Geometry: final body of the model. Coordinates: model frame, mm. Face numbers are marked on the shaded views. A direction names the side the tool comes from. Round coordinates to 2 decimals unless told otherwise and drop trailing zeros. Loops run counter-clockwise (first coordinate to the right, second up) from the corner with the lowest first, then second, coordinate; pieces in that order, holes last. Notation, with made-up numbers: (65, -27.5) -> (110, -27.5) arc R33 ccw to (110, 0.5) -> close; hole circle Ø9 at (18, 65.5). An arc over 180 degrees is marked (long way). Answer in a Markdown table with one row per item.
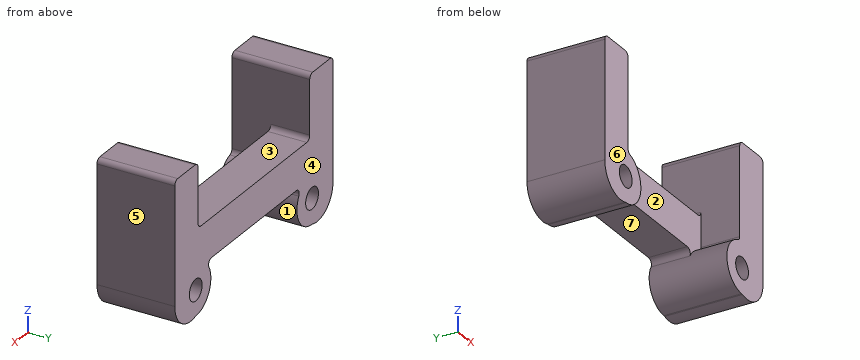
```python
from build123d import *

# Parameters (mm, degrees)
SKETCH1_R           = 1.1
BASE_DEPTH          = 8
BOSS_EXTRUDE2_START = -4
BOSS_EXTRUDE2_DEPTH = 4
FILLET1_R           = 0.5


with BuildPart() as part:
    # Sketch1 → Base (new body)
    with BuildSketch(Plane(origin=(0, 0, 0), x_dir=(1, 0, 0), z_dir=(0, 1, 0))):
        with BuildLine():
            Line((3.6, 0), (3.6, -12.569046516))
            Line((3.6, -12.569046516), (-0.4, -12.569046516))
            Line((-0.4, -12.569046516), (-0.4, -2.569046516))
            ThreePointArc((-0.4, -2.569046516), (-2.592250079, 0.20059793), (0, 2.6))
            ThreePointArc((0, 2.6), (2.464704684, 2.220360331), (3.6, 0))
        make_face()
        with Locations(Location((0, 0, 0), (0, 0, 270))):
            Circle(SKETCH1_R, mode=Mode.SUBTRACT)
    extrude(amount=BASE_DEPTH)

    # Sketch2 → Boss-Extrude2 (add)
    with BuildSketch(Plane(origin=(0, 8, 0), x_dir=(1, 0, 0), z_dir=(0, 1, 0)).offset(BOSS_EXTRUDE2_START)):
        with BuildLine():
            ThreePointArc((-0.4, -2.569046516), (-1.069213935, -2.369975013), (-1.661324773, -2))
            Line((-1.661324773, -2), (-10, -2))
            Line((-10, -2), (-10, -6))
            Line((-10, -6), (-0.4, -6))
            Line((-0.4, -6), (-0.4, -2.569046516))
        make_face()
    extrude(amount=BOSS_EXTRUDE2_DEPTH)

    # Mirror2: part across plane


with BuildPart() as part_1:
    add(part.part)
    add(part.part.mirror(Plane.ZY.offset(10)))

    # Fillet1
    fillet1_edges = [part_1.edges().sort_by_distance(p)[0] for p in [
        (-0.4, 2, 2.569046516),
        (-1.661324773, 6, 2),
        (-0.4, 6, 6),
        (-20, 4, -2.6),
        (-19.6, 2, 2.569046516),
        (-19.6, 4, 12.569046516),
        (-19.6, 6, 6),
        (-23.6, 4, 12.569046516),
        (-18.338675227, 6, 2),
        (3.6, 4, 12.569046516),
        (-0.4, 4, 12.569046516),
        (0, 4, -2.6),
    ]]
    fillet(fillet1_edges, radius=FILLET1_R)


solid = part_1.part
```
Item 1: Set-up query: the marked faces 1, 2, 3 and 4. Return all of +Z, -Z, +X, -X, +Y, -Y with unobstructed straight access to the full face (end or side cutting, diameter ignored); none if empty.
Ans:
| item | result |
|---|---|
| face 1 | -Y |
| face 2 | +Z, -Y |
| face 3 | +Z, +Y, -Y |
| face 4 | +Z, -Z, +X, -X, +Y |
Item 2: First-contact query: P1, Ø2, axis at x = -10.5, y = 5.5, coming from the +Z side; P2, Ø6, axis at x = -10, z = 3.5, coming from the -Y side; P3, Ø5, axis at x = -14.5, z = 10.5, coming from the -Y side; P4, Ø1.2, axis at x = -11, y = 5.5, coming from the -Z side. Flat tips, straight axial feed; report the tip coordinate or a pass-through.
Ans:
| item | result |
|---|---|
| P1 | z = 6 |
| P2 | y = 4 |
| P3 | through |
| P4 | z = 2 |
Item 3: Ray query, L1, parallel to X at y = 6.5, z = -1; L2, parallel to Y at x = -3, z = 5.75; L3, parallel to Z at x = -20, y = 2.5. Return the intervals inside material, ascending.
Ans:
| item | result |
|---|---|
| L1 | -23.41 to -20.46, -19.54 to -17.6, -2.4 to -0.46, 0.46 to 3.41 |
| L2 | 4 to 8 |
| L3 | -2.61 to -1.1, 1.1 to 12.56 |
Item 4: Section query A-A, the plane z = 7.5. Output: boundary loops of the cut face in (x, y).
Ans:
| item | result |
|---|---|
| outline | (-23.6, 0) -> (-19.6, 0) -> (-19.6, 8) -> (-23.6, 8) -> close; (-0.4, 0) -> (3.6, 0) -> (3.6, 8) -> (-0.4, 8) -> close |
Item 5: Mould query, pull axis X, two halves, no side actions, for the marked faces 5, 6 and 7. Classes: released by +X, released by -X, zero draft, split by the parting line, or undercut.
Ans:
| item | result |
|---|---|
| face 5 | released by +X |
| face 6 | zero draft |
| face 7 | undercut |
Item 6: Section query B-B, the plane y = 2. State how many separate pieces and enclosed holes the cut face has, and give its area (3 significant figures).
Ans:
| item | result |
|---|---|
| separate pieces | 2 |
| enclosed holes | 2 |
| area | 128 mm2 |
Item 7: Section query D-D, the plane x = 0.75. Output: boundary loops of the cut face in (y, z).
Ans:
| item | result |
|---|---|
| outline | (0, -2.74) -> (8, -2.74) -> (8, -0.8) -> (0, -0.8) -> close; (0, 0.8) -> (8, 0.8) -> (8, 12.57) -> (0, 12.57) -> close |
Item 8: Section query C-C, the plane z = 3.75. Output: boundary loops of the cut face in (x, y), and give its area (3 significant figures).
Ans:
| item | result |
|---|---|
| outline | (-23.6, 0) -> (-19.6, 0) -> (-19.6, 4) -> (-0.4, 4) -> (-0.4, 0) -> (3.6, 0) -> (3.6, 8) -> (-23.6, 8) -> close |
| area | 141 mm2 |
